Geometry: final body of the model. Coordinates: model frame, mm. Face numbers are marked on the shaded views. Give positions to 0.01 mm unless a question says otherwise; leave off trailing zeros. Loops run counter-clockwise (first coordinate to the right, second up) from the corner with the lowest first, then second, coordinate; pieces in that order, holes last.
1. Draft query along Y for the marked faces 1, 2 and 3. Return one class per face: +Y half, -Y half, draft (parallel to the pull), parting line (faces both ways), or undercut.
2. First-contact query: P1, Ø7, axis at x = 34.925, y = 0, coming from the -Z side; P2, Ø1.5, axis at y = -6, z = 15, coming from the +X side; P3, Ø1.5, axis at x = -2, z = 23.5, coming from the -Y side; P4, Ø12.5, axis at x = -34.925, y = 0, coming from the -Z side. Flat tips, straight axial feed; report the tip coordinate or a pass-through.
3. Section A-A, the plane y = 0. State how many separate pieces and enclosed holes the cut face has, then the cut area to 3 significant figures.
4. Section C-C, the plane z = 43. Output: boundary loops of the cut face in (x, y).
5. Material intervals for line 1 along Z through (x, y) = (29, 3); line 2 along Z through (x, y) = (14, 9); line 3 along Z through (x, y) = (12, -4.5), sorted ascending.
6. Section B-B, the plane z = 12. Output: boundary loops of the cut face in (x, y) (3 decimals), then the cut area to 3 significant figures.
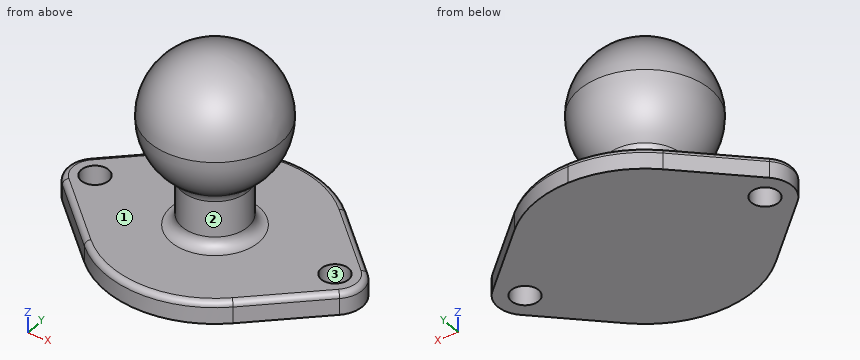
from build123d import *

# Parameters (mm, degrees)
F0_R     = 3.96875
F1_DEPTH = 6.35
F4_DEPTH = 15.2522160579
F5_R     = 1.6002
F6_R     = 3.175


with BuildPart() as f1:
    # F0 (on Top) → F1 (new body)
    with BuildSketch(Plane.XY):
        with BuildLine():
            Line((40.3369318182, 5.8064533276), (21.6477272727, 23.2258133103))
            ThreePointArc((21.6477272727, 23.2258133103), (11.6327754082, 29.5421907837), (0, 31.75))
            ThreePointArc((0, 31.75), (-11.6327754082, 29.5421907837), (-21.6477272727, 23.2258133103))
            Line((-21.6477272727, 23.2258133103), (-40.3369318182, 5.8064533276))
            ThreePointArc((-40.3369318182, 5.8064533276), (-42.8625, 0), (-40.3369318182, -5.8064533276))
            Line((-40.3369318182, -5.8064533276), (-21.6477272727, -23.2258133103))
            ThreePointArc((-21.6477272727, -23.2258133103), (0, -31.75), (21.6477272727, -23.2258133103))
            Line((21.6477272727, -23.2258133103), (40.3369318182, -5.8064533276))
            ThreePointArc((40.3369318182, -5.8064533276), (42.8625, 0), (40.3369318182, 5.8064533276))
        make_face()
        with Locations((-34.925, 0)):
            Circle(F0_R, mode=Mode.SUBTRACT)
        with BuildLine():
            ThreePointArc((9.525, 0), (-6.7351920908, -6.7351920908), (0, 9.525))
            ThreePointArc((0, 9.525), (6.7351920908, 6.7351920908), (9.525, 0))
        make_face(mode=Mode.SUBTRACT)
        with BuildLine():
            ThreePointArc((38.89375, 0), (34.925, -3.96875), (30.95625, 0))
            ThreePointArc((30.95625, 0), (34.925, 3.96875), (38.89375, 0))
        make_face(mode=Mode.SUBTRACT)
        with BuildLine():
            Line((0, 0), (0, 9.525))
            ThreePointArc((0, 9.525), (-6.7351920908, -6.7351920908), (9.525, 0))
            Line((9.525, 0), (0, 0))
        make_face()
        with BuildLine():
            ThreePointArc((9.525, 0), (6.7351920908, 6.7351920908), (0, 9.525))
            Line((0, 9.525), (0, 0))
            Line((0, 0), (9.525, 0))
        make_face()
    extrude(amount=-F1_DEPTH)



with BuildPart() as f3:
    # F2 (on Front) → F3 (revolve)
    with BuildSketch(Plane.XZ):
        with BuildLine():
            Line((0, 50.8), (0, 12.7))
            ThreePointArc((0, 12.7), (13.4703841816, 18.2796158184), (19.05, 31.75))
            ThreePointArc((19.05, 31.75), (13.4703841816, 45.2203841816), (0, 50.8))
        make_face()
    revolve(axis=Axis((0, 0, 25.4), (0, 0, 1)))


with BuildPart() as f1_1:
    add(f1.part)

    add(f3.part)  # F4 merges F3
    # F0 (on Top) → F4 (join, through all)
    with BuildSketch(Plane.XY):
        with BuildLine():
            Line((0, 0), (0, 9.525))
            ThreePointArc((0, 9.525), (-6.7351920908, -6.7351920908), (9.525, 0))
            Line((9.525, 0), (0, 0))
        make_face()
        with BuildLine():
            ThreePointArc((9.525, 0), (6.7351920908, 6.7351920908), (0, 9.525))
            Line((0, 9.525), (0, 0))
            Line((0, 0), (9.525, 0))
        make_face()
    extrude(amount=F4_DEPTH)

    # F5
    f5_edges = [f1_1.edges().sort_by_distance(p)[0] for p in [
        (0, -31.75, 0),
        (42.8625, 0, 0),
        (30.99233, -14.516133, 0),
        (30.99233, 14.516133, 0),
        (0, 31.75, 0),
        (-30.99233, -14.516133, 0),
        (-30.99233, 14.516133, 0),
        (-42.8625, 0, 0),
    ]]
    fillet(f5_edges, radius=F5_R)

    # F6
    f6_edges = [f1_1.edges().sort_by_distance(p)[0] for p in [
        (-9.525, 0, 15.252216),
        (-9.525, 0, 0),
    ]]
    fillet(f6_edges, radius=F6_R)


solid = f1_1.part
Answers below:
1. face 1: draft
1. face 2: parting line
1. face 3: undercut
2. P1: passes through
2. P2: stops at x = 8.69
2. P3: stops at y = -17.41
2. P4: stops at z = -6.35
3. separate pieces: 3
3. enclosed holes: 0
3. area: 1,850 mm2
4. outline: circle Ø30.75 at (0, 0)
5. line 1: z = -6.35 to 0
5. line 2: z = -6.35 to 0, 22.48 to 41.02
5. line 3: z = -6.35 to 0, 17.66 to 45.84
6. outline: circle Ø19.05 at (0, 0)
6. area: 285 mm2
